from build123d import *

# Parameters (mm, degrees)
SKETCH1_R           = 2.125
SKETCH1_R_2         = 1.5
SKETCH1_R_3         = 2.625
BOSS_EXTRUDE1_DEPTH = 2.54
FILLET1_R           = 10
CUT_EXTRUDE2_DEPTH  = 40.369813627
FILLET2_R           = 2


with BuildPart() as part:
    # Sketch1 → Boss-Extrude1 (new body)
    with BuildSketch(Plane(origin=(0, 0, 0), x_dir=(0, 0, -1), z_dir=(1, 0, 0))):
        with BuildLine():
            Line((15, 17.5), (28.675, 17.5))
            ThreePointArc((28.675, 17.5), (33.271194078, 15.596194078), (35.175, 11))
            Line((35.175, 11), (35.175, -3.154825142))
            ThreePointArc((35.175, -3.154825142), (33.366520443, -8.890589505), (28.595201433, -12.551751349))
            Line((28.595201433, -12.551751349), (15, -17.5))
            Line((15, -17.5), (-15, -17.5))
            Line((-15, -17.5), (-28.595201433, -12.551751349))
            ThreePointArc((-28.595201433, -12.551751349), (-33.366520443, -8.890589505), (-35.175, -3.154825142))
            Line((-35.175, -3.154825142), (-35.175, 11))
            ThreePointArc((-35.175, 11), (-33.271194078, 15.596194078), (-28.675, 17.5))
            Line((-28.675, 17.5), (-15, 17.5))
            Line((-15, 17.5), (15, 17.5))
        make_face()
        with Locations((28.675, 11)):
            Circle(SKETCH1_R, mode=Mode.SUBTRACT)
        with Locations(Location((-28.675, 11, 0), (0, 0, 180))):
            Circle(SKETCH1_R, mode=Mode.SUBTRACT)
        with Locations((28, 2.5)):
            Circle(SKETCH1_R_2, mode=Mode.SUBTRACT)
        with Locations(Location((-28, 2.5, 0), (0, 0, 180))):
            Circle(SKETCH1_R_2, mode=Mode.SUBTRACT)
        with Locations((28.675, -7)):
            Circle(SKETCH1_R_3, mode=Mode.SUBTRACT)
        with Locations(Location((-28.675, -7, 0), (0, 0, 180))):
            Circle(SKETCH1_R_3, mode=Mode.SUBTRACT)
    extrude(amount=BOSS_EXTRUDE1_DEPTH)

    # Fillet1
    fillet1_edges = [part.edges().sort_by_distance(p)[0] for p in [
        (1.27, -17.5, -15),
        (1.27, -17.5, 15),
    ]]
    fillet(fillet1_edges, radius=FILLET1_R)

    # Sketch2 → Cut-Extrude2 (cut, through all)
    with BuildSketch(Plane(origin=(0, 0, 0), x_dir=(0, 0, -1), z_dir=(1, 0, 0))):
        with BuildLine():
            ThreePointArc((-23.774426054, 12.5), (-23.583197925, 11.582388729), (-23.562289313, 10.645296699))
            Line((-23.562289313, 10.645296699), (-1.5, 2.181994783))
            Line((-1.5, 2.181994783), (-1.5, 12.5))
            Line((-1.5, 12.5), (-23.774426054, 12.5))
        make_face()
        with BuildLine():
            ThreePointArc((-23.040869369, 7.232113781), (-24.495524174, 6.805676348), (-24.469315886, 5.29003041))
            ThreePointArc((-24.469315886, 5.29003041), (-23.690537785, 1.204416959), (-26.593153981, -1.774433796))
            ThreePointArc((-26.593153981, -1.774433796), (-24.964789293, -2.77212092), (-23.764069674, -4.257120431))
            Line((-23.764069674, -4.257120431), (-5.019125542, 0.318803158))
            Line((-5.019125542, 0.318803158), (-23.040869369, 7.232113781))
        make_face()
        with BuildLine():
            Line((23.774426054, 12.5), (1.5, 12.5))
            Line((1.5, 12.5), (1.5, 2.181994783))
            Line((1.5, 2.181994783), (23.562289313, 10.645296699))
            ThreePointArc((23.562289313, 10.645296699), (23.583197925, 11.582388729), (23.774426054, 12.5))
        make_face()
        with BuildLine():
            Line((-1.5, -12.5), (-1.5, -1.91022003))
            Line((-1.5, -1.91022003), (-23.052616211, -7.171538721))
            ThreePointArc((-23.052616211, -7.171538721), (-23.169671761, -8.15411697), (-23.457097153, -9.100979506))
            Line((-23.457097153, -9.100979506), (-14.94683091, -12.198463104))
            ThreePointArc((-14.94683091, -12.198463104), (-14.104971081, -12.424038765), (-13.236730193, -12.5))
            Line((-13.236730193, -12.5), (-1.5, -12.5))
        make_face()
        with BuildLine():
            Line((23.052616211, -7.171538721), (1.5, -1.91022003))
            Line((1.5, -1.91022003), (1.5, -12.5))
            Line((1.5, -12.5), (13.236730193, -12.5))
            ThreePointArc((13.236730193, -12.5), (14.104971081, -12.424038765), (14.94683091, -12.198463104))
            Line((14.94683091, -12.198463104), (23.457097153, -9.100979506))
            ThreePointArc((23.457097153, -9.100979506), (23.169671761, -8.15411697), (23.052616211, -7.171538721))
        make_face()
        with BuildLine():
            Line((23.040869369, 7.232113781), (5.019125542, 0.318803158))
            Line((5.019125542, 0.318803158), (23.764069674, -4.257120431))
            ThreePointArc((23.764069674, -4.257120431), (24.964789293, -2.77212092), (26.593153981, -1.774433796))
            ThreePointArc((26.593153981, -1.774433796), (23.690537785, 1.204416959), (24.469315886, 5.29003041))
            ThreePointArc((24.469315886, 5.29003041), (24.495524174, 6.805676348), (23.040869369, 7.232113781))
        make_face()
    extrude(amount=CUT_EXTRUDE2_DEPTH, mode=Mode.SUBTRACT)

    # Fillet2
    # the kernel refuses this fillet: 2 mm, written as the material it adds along each edge
    with BuildSketch(Plane(origin=(0, -12.5, -1.5), x_dir=(0, 0, -1), z_dir=(1, 0, 0)), Plane(origin=(0, 12.5, -1.5), x_dir=(0, -1, 0), z_dir=(1, 0, 0))) as fillet2_piece_1:
        with BuildLine():
            CenterArc((FILLET2_R, FILLET2_R), FILLET2_R, 180, 90)
            Line((0, FILLET2_R), (0, 0))
            Line((0, 0), (FILLET2_R, 0))
        make_face()
    extrude(amount=2.54)
    with BuildSketch(Plane(origin=(0, -12.5, 1.5), x_dir=(0, 0, 1), z_dir=(1, 0, 0)), Plane(origin=(0, 12.5, 1.5), x_dir=(0, -1, 0), z_dir=(1, 0, 0))) as fillet2_piece_2:
        with BuildLine():
            CenterArc((FILLET2_R, -FILLET2_R), FILLET2_R, 90, 90)
            Line((0, -FILLET2_R), (0, 0))
            Line((0, 0), (FILLET2_R, 0))
        make_face()
    extrude(amount=2.54)
    with BuildSketch(Plane(origin=(0, -1.91022003, -1.5), x_dir=(0, -1, 0), z_dir=(1, 0, 0)), Plane(origin=(0, -1.91022003, 1.5), x_dir=(0, -0.23715115410902912, 0.9714727634394881), z_dir=(1, 0, 0))) as fillet2_piece_3:
        with BuildLine():
            CenterArc((FILLET2_R * 1.27348001989, FILLET2_R), FILLET2_R, 166.281540054, 103.718459946)
            Line((FILLET2_R * 0.302007256452, FILLET2_R * 1.23715115411), (0, 0))
            Line((0, 0), (FILLET2_R * 1.27348001989, 0))
        make_face()
    extrude(amount=2.54)
    with BuildSketch(Plane(origin=(0, -9.100979506, -23.457097153), x_dir=(0, 0.9698771558526914, 0.24359454541326273), z_dir=(1, 0, 0))) as fillet2_piece_4:
        with BuildLine():
            CenterArc((1.805861593, 1.981337572), FILLET2_R, 185.90120906, 76.265486652)
            Line((-0.183539703, 1.775710517), (0, 0))
            ThreePointArc((0, 0), (0.766639355, 0.05248808), (1.533278711, 0))
        make_face()
    extrude(amount=2.54)
    with BuildSketch(Plane(origin=(0, -7.171538721, -23.052616211), x_dir=(0, -0.991038367867246, -0.13357751837425885), z_dir=(1, 0, 0)), Plane(origin=(0, -4.257120431, 23.764069674), x_dir=(0, 0.8180162943485203, 0.5751950470756115), z_dir=(1, 0, 0))) as fillet2_piece_5:
        with BuildLine():
            CenterArc((1.368631059, -1.989301963), FILLET2_R, 95.928822705, 62.676344636)
            Line((-0.493546379, -1.259716335), (0, 0))
            ThreePointArc((0, 0), (0.581022619, -0.03008823), (1.162045239, 0))
        make_face()
    extrude(amount=2.54)
    with BuildSketch(Plane(origin=(0, 2.181994783, -1.5), x_dir=(0, 0.3581607437996355, -0.9336599389504147), z_dir=(1, 0, 0)), Plane(origin=(0, 2.181994783, 1.5), x_dir=(0, 1, 0), z_dir=(1, 0, 0))) as fillet2_piece_6:
        with BuildLine():
            CenterArc((FILLET2_R * 1.45466318853, FILLET2_R), FILLET2_R, 159.012716108, 110.987283892)
            Line((FILLET2_R * 0.521003249583, FILLET2_R * 1.3581607438), (0, 0))
            Line((0, 0), (FILLET2_R * 1.45466318853, 0))
        make_face()
    extrude(amount=2.54)
    with BuildSketch(Plane(origin=(0, 10.645296699, -23.562289313), x_dir=(0, -0.3581607437996529, 0.9336599389504079), z_dir=(1, 0, 0))) as fillet2_piece_7:
        with BuildLine():
            CenterArc((1.305521848, -2), FILLET2_R, 90, 60.578668933)
            ThreePointArc((-0.436540129, -1.01754386), (-0.190709987, -0.520595577), (0, 0))
            Line((0, 0), (1.305521848, 0))
        make_face()
    extrude(amount=2.54)
    with BuildSketch(Plane(origin=(0, 12.5, -23.774426054), x_dir=(0, 0, 1), z_dir=(1, 0, 0))) as fillet2_piece_8:
        with BuildLine():
            CenterArc((2.206860542, 2), FILLET2_R, 184.024063889, 85.975936111)
            ThreePointArc((0.211791212, 1.859649123), (0.191509232, 0.92007422), (0, 0))
            Line((0, 0), (2.206860542, 0))
        make_face()
    extrude(amount=2.54)
    with BuildSketch(Plane(origin=(0, -7.171538721, 23.052616211), x_dir=(0, -0.9910383678672416, 0.13357751837428994), z_dir=(1, 0, 0))) as fillet2_piece_9:
        with BuildLine():
            CenterArc((1.368631059, 1.989301963), FILLET2_R, 201.394832659, 62.676344636)
            Line((-0.493546379, 1.259716335), (0, 0))
            ThreePointArc((0, 0), (0.581022619, 0.03008823), (1.162045239, 0))
        make_face()
    extrude(amount=2.54)
    with BuildSketch(Plane(origin=(0, -9.100979506, 23.457097153), x_dir=(0, -0.342020143325639, -0.9396926207859192), z_dir=(1, 0, 0))) as fillet2_piece_10:
        with BuildLine():
            CenterArc((1.785170766, 2), FILLET2_R, 193.734513348, 76.265486652)
            ThreePointArc((-0.157641792, 1.525153327), (-0.026610969, 0.767973148), (0, 0))
            Line((0, 0), (1.785170766, 0))
        make_face()
    extrude(amount=2.54)
    with BuildSketch(Plane(origin=(0, 0.318803158, -5.019125542), x_dir=(0, -0.23715115410902946, -0.971472763439488), z_dir=(1, 0, 0)), Plane(origin=(0, 0.318803158, 5.019125542), x_dir=(0, 0.3581607437996354, 0.9336599389504147), z_dir=(1, 0, 0))) as fillet2_piece_11:
        with BuildLine():
            CenterArc((FILLET2_R * 3.20022614882, FILLET2_R), FILLET2_R, 124.705743839, 145.294256161)
            Line((FILLET2_R * 2.63086420922, FILLET2_R * 1.82208696726), (0, 0))
            Line((0, 0), (FILLET2_R * 3.20022614882, 0))
        make_face()
    extrude(amount=2.54)
    with BuildSketch(Plane(origin=(0, -4.257120431, -23.764069674), x_dir=(0, 0.23715115410907214, 0.9714727634394775), z_dir=(1, 0, 0))) as fillet2_piece_12:
        with BuildLine():
            CenterArc((1.352949842, -2), FILLET2_R, 90, 62.676344636)
            ThreePointArc((-0.423905752, -1.081967213), (-0.183938065, -0.551959577), (0, 0))
            Line((0, 0), (1.352949842, 0))
        make_face()
    extrude(amount=2.54)
    with BuildSketch(Plane(origin=(0, -1.774433796, -26.593153981), x_dir=(0, 0.5517747839578403, 0.8339931581183857), z_dir=(1, 0, 0))) as fillet2_piece_13:
        with BuildLine():
            CenterArc((2.89721625, 1.929382533), FILLET2_R, 170.336114641, 84.3929753)
            ThreePointArc((0.925597299, 2.265118609), (0.587459761, 1.081618931), (0, 0))
            ThreePointArc((0, 0), (1.18522483, 0.158889301), (2.370449659, 0))
        make_face()
    extrude(amount=2.54)
    with BuildSketch(Plane(origin=(0, -1.774433796, 26.593153981), x_dir=(0, -0.5633055097989954, -0.826248692967253), z_dir=(1, 0, 0))) as fillet2_piece_14:
        with BuildLine():
            CenterArc((2.881946095, 1.95211825), FILLET2_R, 173.04447146, 84.3929753)
            ThreePointArc((0.896665206, 2.194316088), (0.595415815, 1.037055309), (0, 0))
            ThreePointArc((0, 0), (1.223467682, 0.134667421), (2.446935364, 0))
        make_face()
    extrude(amount=2.54)
    with BuildSketch(Plane(origin=(0, 12.5, 23.774426054), x_dir=(0, -0.9935772054285649, -0.11315624972913957), z_dir=(1, 0, 0))) as fillet2_piece_15:
        with BuildLine():
            CenterArc((2.236874473, 1.966373831), FILLET2_R, 173.502708243, 85.975936111)
            Line((0.249720063, 2.19268633), (0, 0))
            ThreePointArc((0, 0), (0.935835239, 0.086167059), (1.871670478, 0))
        make_face()
    extrude(amount=2.54)
    with BuildSketch(Plane(origin=(0, 10.645296699, 23.562289313), x_dir=(0, -0.35816074379962426, -0.9336599389504189), z_dir=(1, 0, 0))) as fillet2_piece_16:
        with BuildLine():
            CenterArc((1.305521848, 2), FILLET2_R, 209.421331067, 60.578668933)
            ThreePointArc((-0.436540129, 1.01754386), (-0.190709987, 0.520595577), (0, 0))
            Line((0, 0), (1.305521848, 0))
        make_face()
    extrude(amount=2.54)


solid = part.part
Source: CAD feature listing. Evaluate the final solid. Frame: model axes, mm. A direction names the side the tool comes from. Coordinates: 2 decimals unless noted, no trailing zeros. Loops run counter-clockwise (first coordinate to the right, second up) from the corner with the lowest first, then second, coordinate; pieces in that order, holes last. Notation, with made-up numbers: (40, 35) -> (51, 35) arc R18 ccw to (51, 57) -> close; hole circle Ø5 at (-40, 40). An arc over 180 degrees is marked (long way). Answer in a Markdown table with one row per item. Add a question column.
Q1. Section A-A on z = 14. Return the cut outline in (x, y).
Q2. Reachability of faces 4 (the face through (2.54, 1, -1)), 5 (the face through (1.25, -10.94, 18.41)) from +Z, -Z, +X, -X, +Y, -Y: full face, straight path, thin tool, end or side. Return the list, or none.
Q3. Section B-B on x = 0.5. Give the number of separate pieces and of enclosed holes in the cut face, and give its area (3 significant figures).
Q4. Ray query, line 1 along Y through (x, z) = (1.5, 19.5); line 2 along Y through (x, z) = (0.35, -3.5); line 3 along Y through (x, z) = (1.45, -19). Return the intervals inside material, ascending.
Q5. Contact query for a flat-ended pin moving along its axis: pin 1 Ø0.8 at (x, y) = (2, -8.5) entering from -Z. Output: stop coordinate, or through.
Q6. Pull-direction query (Y, two-part tool) for faces 1 (the face through (1.252, -1.798, 25.112)), 2 (the face through (1, 17.5, 0)), 3 (the face through (0, 1, -1)); classes: pulls with the +Y half, pulls with the -Y half, needs draft (parallel to the pull), parting line crosses it, or undercut.
Computed values:
| question | item | result |
|---|---|---|
| 1 | outline | (0, -17.47) -> (2.54, -17.47) -> (2.54, -12.44) -> (0, -12.44) -> close; (0, -4.96) -> (2.54, -4.96) -> (2.54, -1.87) -> (0, -1.87) -> close; (0, 3.76) -> (2.54, 3.76) -> (2.54, 6.98) -> (0, 6.98) -> close; (0, 12.5) -> (2.54, 12.5) -> (2.54, 17.5) -> (0, 17.5) -> close |
| 2 | face 4 | +Z, -Z, +X, +Y, -Y |
| 2 | face 5 | +X, -X |
| 3 | separate pieces | 1 |
| 3 | enclosed holes | 12 |
| 3 | area | 1,410 mm^2 |
| 4 | line 1 | y = -15.86 to -10.54, -6.3 to -3.22, 5.87 to 9.09, 12.5 to 17.5 |
| 4 | line 2 | y = -17.5 to -12.5, -2.46 to 3.09, 12.5 to 17.5 |
| 4 | line 3 | y = -16.04 to -10.72, -6.18 to -3.09, 5.68 to 8.9, 12.5 to 17.5 |
| 5 | pin 1 | stops at z = -33.87 |
| 6 | face 1 | undercut |
| 6 | face 2 | pulls with the +Y half |
| 6 | face 3 | needs draft |
